```python
from build123d import *

# Parameters (mm, degrees)
BOSS_EXTRUDE1_DEPTH = 84.074
SKETCH3_W           = 76.581
SKETCH3_H           = 76.581
BOSS_EXTRUDE2_DEPTH = 31.75
SKETCH_D_R          = 15.875
BOSS_EXTRUDE3_DEPTH = 69.85
CUT_EXTRUDE1_DEPTH  = 35.56
FILLET1_R           = 6.35
FILLET2_R           = 1.27
KEYWAY_START        = 12.3698
KEYWAY_DEPTH        = 67.8782
CHAMFER1_SIZE       = 0.381
SKETCH7_R           = 15.875
CUT_EXTRUDE3_DEPTH  = 186.674


with BuildPart() as part:
    # L,M → Boss-Extrude1 (new body)
    with BuildSketch(Plane.XY):
        Polygon((-100.076, 68.326), (100.076, 68.326), (100.076, 207.077403609), (84.201, 222.952403609), (84.201, 288.603596391), (37.778596391, 335.026), (-37.778596391, 335.026), (-84.201, 288.603596391), (-84.201, 222.952403609), (-100.076, 207.077403609), align=None)
    extrude(amount=BOSS_EXTRUDE1_DEPTH)

    # Sketch3 → Boss-Extrude2 (add)
    with BuildSketch(Plane.XY.offset(84.074)):
        with Locations((0, 255.778)):
            Rectangle(SKETCH3_W, SKETCH3_H)
    extrude(amount=BOSS_EXTRUDE2_DEPTH)

    # D → Boss-Extrude3 (add)
    with BuildSketch(Plane.XY.offset(115.824)):
        with Locations((0, 255.778)):
            Circle(SKETCH_D_R)
    extrude(amount=BOSS_EXTRUDE3_DEPTH)

    # Sketch5 → Cut-Extrude1 (cut)
    with BuildSketch(Plane.XY.offset(84.074)):
        Polygon((100.076, 114.748403609), (53.653596391, 68.326), (100.076, 68.326), align=None)
        Polygon((-100.076, 68.326), (-100.076, 114.748403609), (-53.653596391, 68.326), align=None)
    extrude(amount=-CUT_EXTRUDE1_DEPTH, mode=Mode.SUBTRACT)

    # Fillet1
    fillet1_edges = [part.edges().sort_by_distance(p)[0] for p in [
        (-38.2905, 294.0685, 99.949),
        (-38.2905, 217.4875, 99.949),
        (38.2905, 217.4875, 99.949),
        (38.2905, 294.0685, 99.949),
    ]]
    fillet(fillet1_edges, radius=FILLET1_R)

    # Fillet2
    fillet2_edges = [part.edges().sort_by_distance(p)[0] for p in [
        (100.076, 160.912903609, 84.074),
        (76.864798195, 91.537201805, 84.074),
        (92.1385, 215.014903609, 84.074),
        (84.201, 255.778, 84.074),
        (60.989798195, 311.814798195, 84.074),
        (0, 335.026, 84.074),
        (0, 68.326, 84.074),
        (-60.989798195, 311.814798195, 84.074),
        (-84.201, 255.778, 84.074),
        (-92.1385, 215.014903609, 84.074),
        (-100.076, 160.912903609, 84.074),
        (-76.864798195, 91.537201805, 84.074),
        (0, 217.4875, 84.074),
        (-38.2905, 255.778, 84.074),
        (38.2905, 255.778, 84.074),
        (0, 294.0685, 84.074),
        (-36.430628061, 219.347371939, 84.074),
        (36.430628061, 219.347371939, 84.074),
        (-36.430628061, 292.208628061, 84.074),
        (36.430628061, 292.208628061, 84.074),
    ]]
    fillet(fillet2_edges, radius=FILLET2_R)

    # Sketch6 → Keyway (cut, through all)
    with BuildSketch(Plane(origin=(0, 255.778, 0), x_dir=(-1, 0, 0), z_dir=(0, 1, 0)).offset(KEYWAY_START)):
        with BuildLine():
            Line((3.175, 185.674), (3.175, 120.904))
            ThreePointArc((3.175, 120.904), (0, 117.729), (-3.175, 120.904))
            Line((-3.175, 120.904), (-3.175, 185.674))
            ThreePointArc((-3.175, 185.674), (0, 188.849), (3.175, 185.674))
        make_face()
    extrude(amount=KEYWAY_DEPTH, mode=Mode.SUBTRACT)

    # Chamfer1
    chamfer1_edges = [part.edges().sort_by_distance(p)[0] for p in [
        (-10.040231571, 243.481277876, 185.674),
    ]]
    chamfer(chamfer1_edges, length=CHAMFER1_SIZE)

    # Sketch7 → Cut-Extrude3 (cut, through all)
    with BuildSketch(Plane(origin=(0, 0, 0), x_dir=(-1, 0, 0), z_dir=(0, 0, -1))):
        with Locations((0, 136.652)):
            Circle(SKETCH7_R)
    extrude(amount=-CUT_EXTRUDE3_DEPTH, mode=Mode.SUBTRACT)


solid = part.part
```
The model under review builds one solid part; all positions refer to its coordinate system, in mm. A direction names the side the tool comes from. Coordinates: 2 decimals unless noted, no trailing zeros. Order: outer loops, then holes, each group sorted by start corner. A loop starts at its lowest first (then second) coordinate and runs counter-clockwise, first axis right, second up. Notation, with made-up numbers: (51, 48) -> (69, 48) arc R21 ccw to (69, 79) -> close; hole circle Ø11 at (-39, 11). An arc over 180 degrees is marked (long way). Answer in a Markdown table with one row per item. Add a question column.
Item 1: We need section D-D on y = 125. Write out the cut boundary in (x, z), plus the area to 3 significant figures.
Item 2: We need section B-B on z = 109. Write out the cut boundary in (x, y), plus the area to 3 significant figures.
Item 3: Clearance check with flat-ended pins moving along their axes: pin 1 (1.6 mm diameter, centred on y = 269.5, z = 146, fed in from -X); pin 2 (15 mm diameter, centred on x = -4.5, z = 102.5, fed in from -Y); pin 3 (24.5 mm diameter, centred on x = -12.5, z = 97.5, fed in from +Y). State where each tip first meets the part, or that it passes through.
Item 4: Mouldability with a two-part tool opening along Y and no side actions: class faces 6 (the flat face through (92.25, 214.904, 40.822)), 7 (the cylindrical face through (76.27, 91.48, 83.71)), 8 (the cylindrical face through (3.441, 121.155, 41.448)), 9 (the flat face through (-38.29, 255, 100)) as +Y half, -Y half, draft (parallel to the pull), parting line (faces both ways), or undercut.
Item 5: To check wall thickness, follow probe 1 along Y at (x, z) = (0, 56); probe 2 along Z at (x, y) = (71.5, 167.5); probe 3 along X at (y, z) = (263, 9.5). State the ranges of each line that lie inside material, in increasing order.
Item 6: We need section C-C on x = 25. Write out the cut boundary in (y, z), plus the area to 3 significant figures.
Item 7: We need section A-A on x = 0. Write out the cut boundary in (y, z), plus the area to 3 significant figures.
Item 8: Machinability: for faces 1 (the flat face through (-1, 239, 115.824)), 2 (the flat face through (87, 82, 48.514)), 3 (the flat face through (-87, 82, 48.514)), 4 (the cylindrical face through (-36.48, 292.16, 100.8)), 5 (the flat face through (0, 256, 185.674)), which of the approach directions +Z, -Z, +X, -X, +Y, -Y give a long, thin tool a straight path to every point of the face, cutting with its end or side? Answer none if there is none.
Final values:
| question | item | result |
|---|---|---|
| 1 | outline | (-100.08, 0) -> (-10.78, 0) -> (-10.78, 84.07) -> (-98.81, 84.07) arc R1.27 ccw to (-100.08, 82.8) -> close; (10.78, 0) -> (100.08, 0) -> (100.08, 82.8) arc R1.27 ccw to (98.81, 84.07) -> (10.78, 84.07) -> close |
| 1 | area | 15,000 mm2 |
| 2 | outline | (-38.29, 223.84) arc R6.35 ccw to (-31.94, 217.49) -> (31.94, 217.49) arc R6.35 ccw to (38.29, 223.84) -> (38.29, 287.72) arc R6.35 ccw to (31.94, 294.07) -> (-31.94, 294.07) arc R6.35 ccw to (-38.29, 287.72) -> close |
| 2 | area | 5,830 mm2 |
| 3 | pin 1 | stops at x = -9.22 |
| 3 | pin 2 | stops at y = 217.49 |
| 3 | pin 3 | stops at y = 294.07 |
| 4 | face 6 | +Y half |
| 4 | face 7 | -Y half |
| 4 | face 8 | undercut |
| 4 | face 9 | draft |
| 5 | probe 1 | y = 68.33 to 120.78, 152.53 to 335.03 |
| 5 | probe 2 | z = 0 to 84.07 |
| 5 | probe 3 | x = -84.2 to 84.2 |
| 6 | outline | (68.33, 0) -> (335.03, 0) -> (335.03, 82.8) arc R1.27 ccw to (333.76, 84.07) -> (295.34, 84.07) arc R1.27 cw to (294.07, 85.34) -> (294.07, 115.82) -> (217.49, 115.82) -> (217.49, 85.34) arc R1.27 cw to (216.22, 84.07) -> (69.6, 84.07) arc R1.27 ccw to (68.33, 82.8) -> close |
| 6 | area | 24,900 mm2 |
| 7 | outline | (68.33, 0) -> (120.78, 0) -> (120.78, 84.07) -> (69.6, 84.07) arc R1.27 ccw to (68.33, 82.8) -> close; (152.53, 0) -> (335.03, 0) -> (335.03, 82.8) arc R1.27 ccw to (333.76, 84.07) -> (295.34, 84.07) arc R1.27 cw to (294.07, 85.34) -> (294.07, 115.82) -> (271.65, 115.82) -> (271.65, 117.73) -> (268.15, 117.73) -> (268.15, 185.67) -> (240.28, 185.67) -> (239.9, 185.29) -> (239.9, 115.82) -> (217.49, 115.82) -> (217.49, 85.34) arc R1.27 cw to (216.22, 84.07) -> (152.53, 84.07) -> close |
| 7 | area | 24,200 mm2 |
| 8 | face 1 | +Z |
| 8 | face 2 | +Z, +X, -Y |
| 8 | face 3 | +Z, -X, -Y |
| 8 | face 4 | +Z, -X, +Y |
| 8 | face 5 | +Z, +X, -X, +Y, -Y |
